```python
from build123d import *

# Parameters (mm, degrees)
SKETCH1_R           = 4
BOSS_EXTRUDE1_DEPTH = 235
CUT_EXTRUDE1_DEPTH  = 7.5
SKETCH3_R           = 4
SKETCH3_R_2         = 3.5
CUT_EXTRUDE2_DEPTH  = 1


with BuildPart() as part:
    # Sketch1 → Boss-Extrude1 (new body)
    with BuildSketch(Plane.XY):
        Circle(SKETCH1_R)
    extrude(amount=BOSS_EXTRUDE1_DEPTH)

    # Sketch2 → Cut-Extrude1 (cut)
    with BuildSketch(Plane.XY.offset(235)):
        with BuildLine():
            Line((3.122498999, 2.5), (-3.122498999, 2.5))
            ThreePointArc((-3.122498999, 2.5), (0, 4), (3.122498999, 2.5))
        make_face()
    extrude(amount=-CUT_EXTRUDE1_DEPTH, mode=Mode.SUBTRACT)

    # Sketch3 → Cut-Extrude2 (cut)
    with BuildSketch(Plane.XY.offset(233.75)):
        Circle(SKETCH3_R)
        Circle(SKETCH3_R_2, mode=Mode.SUBTRACT)
    extrude(amount=-CUT_EXTRUDE2_DEPTH, mode=Mode.SUBTRACT)


solid = part.part
```
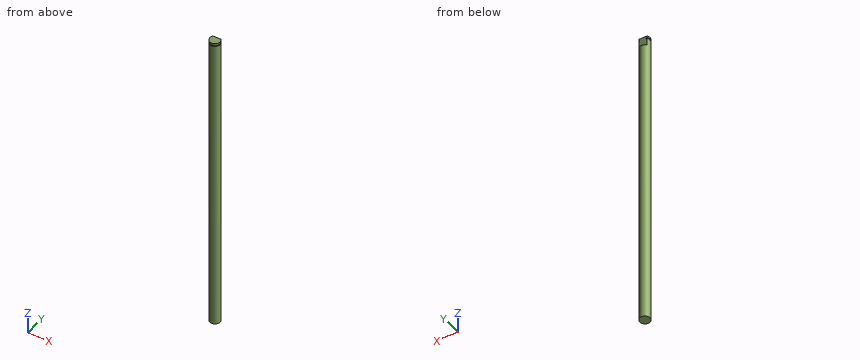
Source: CAD feature listing. Evaluate the final solid. Frame: model axes, mm. Coordinates: 2 decimals unless noted, no trailing zeros. Loops run counter-clockwise (first coordinate to the right, second up) from the corner with the lowest first, then second, coordinate; pieces in that order, holes last. Notation, with made-up numbers: M 77.5,48 L 130.5,48 A21 cw 130.5,80 Z; hole C -13.75,46.5 d6. An arc over 180 degrees is marked long. Put each result on its own line as item: value. Start each with the question number.
1) Cut plane C-C on y = 1.25. Return the cut outline in (x, z).
2) Cut plane A-A on x = 1. Return the cut outline in (y, z), then the cut area to 3 significant figures.
3) Cut plane B-B on z = 66.5. Return the cut outline in (x, y), then the cut area to 3 significant figures.
4) Contact query for flat-ended pins moving along their axis: pin 1 Ø0.8 at (x, y) = (-1.5, 3.5) entering from +Z; pin 2 Ø1 at (y, z) = (-1.5, 188) entering from -X; pin 3 Ø3 at (x, z) = (1, 230) entering from +Y. Output: stop coordinate, or through.
5) Ray query, L1, parallel to Z at x = -3.5, y = -0.5; L2, parallel to Y at x = -0.25, z = 35; L3, parallel to X at y = -2.5, z = 125.5. Return the intervals inside material, ascending. Write a range as from..to.
The answers:
1. outline: M -3.8,0 L 3.8,0 L 3.8,232.75 L 3.27,232.75 L 3.27,233.75 L 3.8,233.75 L 3.8,235 L -3.8,235 L -3.8,233.75 L -3.27,233.75 L -3.27,232.75 L -3.8,232.75 Z
2. outline: M -3.87,0 L 3.87,0 L 3.87,227.5 L 2.5,227.5 L 2.5,235 L -3.87,235 L -3.87,233.75 L -3.35,233.75 L -3.35,232.75 L -3.87,232.75 Z
2. area: 1,810 mm²
3. outline: C 0,0 d8
3. area: 50.3 mm²
4. pin 1: stops at z = 227.5
4. pin 2: stops at x = -3.87
4. pin 3: stops at y = 2.5
5. L1: z = 0..232.75, 233.75..235
5. L2: y = -3.99..3.99
5. L3: x = -3.12..3.12
